```python
from build123d import *

# Parameters (mm, degrees)
SKETCH1_R           = 0.9
SKETCH1_R_2         = 0.65
BOSS_EXTRUDE1_DEPTH = 220
SKETCH2_R           = 0.9
SKETCH2_R_2         = 0.65
CUT_EXTRUDE1_DEPTH  = 6
SKETCH1_3_R         = 0.65
BOSS_EXTRUDE2_DEPTH = 5
FILLET1_R           = 3
FILLET2_R           = 1


with BuildPart() as part:
    # Sketch1 → Boss-Extrude1 (new body)
    # profile 1 of 7: a face of its own
    with BuildSketch(Plane(origin=(-29.212578399, 0, 0), x_dir=(0, 0, -1), z_dir=(1, 0, 0))):
        with BuildLine():
            ThreePointArc((7.945170891, 34.240487163), (7.203959388, 34.412879785), (6.445170891, 34.470791156))
            Line((6.445170891, 34.470791156), (4.445170891, 34.470791156))
            Line((4.445170891, 34.470791156), (4.445170891, 27.470791156))
            Line((4.445170891, 27.470791156), (11.445170891, 27.470791156))
            Line((11.445170891, 27.470791156), (11.445170891, 29.470791156))
            ThreePointArc((11.445170891, 29.470791156), (11.38725952, 30.229579652), (11.214866898, 30.970791156))
            Line((11.214866898, 30.970791156), (7.945170891, 30.970791156))
            Line((7.945170891, 30.970791156), (7.945170891, 34.240487163))
        make_face()
        with Locations((9.695170891, 29.220791156)):
            Circle(SKETCH1_R, mode=Mode.SUBTRACT)
        with Locations((6.195170891, 32.720791156)):
            Circle(SKETCH1_R, mode=Mode.SUBTRACT)
    # profile 2 of 7: a face of its own
    with BuildSketch(Plane(origin=(-29.212578399, 0, 0), x_dir=(0, 0, -1), z_dir=(1, 0, 0))):
        with BuildLine():
            Line((11.445170891, 29.470791156), (11.445170891, 30.970791156))
            Line((11.445170891, 30.970791156), (11.214866898, 30.970791156))
            ThreePointArc((11.214866898, 30.970791156), (11.38725952, 30.229579652), (11.445170891, 29.470791156))
        make_face()
    # profile 3 of 7: a face of its own
    with BuildSketch(Plane(origin=(-29.212578399, 0, 0), x_dir=(0, 0, -1), z_dir=(1, 0, 0))):
        with BuildLine():
            Line((7.945170891, 34.240487163), (7.945170891, 34.470791156))
            Line((7.945170891, 34.470791156), (6.445170891, 34.470791156))
            ThreePointArc((6.445170891, 34.470791156), (7.203959388, 34.412879785), (7.945170891, 34.240487163))
        make_face()
    # profile 4 of 7: a face of its own
    with BuildSketch(Plane(origin=(-29.212578399, 0, 0), x_dir=(0, 0, -1), z_dir=(1, 0, 0))):
        with Locations((6.195170891, 32.720791156)):
            Circle(SKETCH1_R)
        with Locations((6.195170891, 32.720791156)):
            Circle(SKETCH1_R_2, mode=Mode.SUBTRACT)
    # profile 5 of 7: a face of its own
    with BuildSketch(Plane(origin=(-29.212578399, 0, 0), x_dir=(0, 0, -1), z_dir=(1, 0, 0))):
        with Locations((6.195170891, 32.720791156)):
            Circle(SKETCH1_R_2)
    # profile 6 of 7: a face of its own
    with BuildSketch(Plane(origin=(-29.212578399, 0, 0), x_dir=(0, 0, -1), z_dir=(1, 0, 0))):
        with Locations((9.695170891, 29.220791156)):
            Circle(SKETCH1_R)
        with Locations((9.695170891, 29.220791156)):
            Circle(SKETCH1_R_2, mode=Mode.SUBTRACT)
    # profile 7 of 7: a face of its own
    with BuildSketch(Plane(origin=(-29.212578399, 0, 0), x_dir=(0, 0, -1), z_dir=(1, 0, 0))):
        with Locations((9.695170891, 29.220791156)):
            Circle(SKETCH1_R_2)
    extrude(amount=BOSS_EXTRUDE1_DEPTH)

    # Sketch2 → Cut-Extrude1 (cut)
    # profile 1 of 4: a face of its own
    with BuildSketch(Plane(origin=(190.787421601, 0, 0), x_dir=(0, 0, -1), z_dir=(1, 0, 0))):
        with Locations((6.195170891, 32.720791156)):
            Circle(SKETCH2_R)
        with Locations((6.195170891, 32.720791156)):
            Circle(SKETCH2_R_2, mode=Mode.SUBTRACT)
    # profile 2 of 4: a face of its own
    with BuildSketch(Plane(origin=(190.787421601, 0, 0), x_dir=(0, 0, -1), z_dir=(1, 0, 0))):
        with Locations((6.195170891, 32.720791156)):
            Circle(SKETCH2_R_2)
    # profile 3 of 4: a face of its own
    with BuildSketch(Plane(origin=(190.787421601, 0, 0), x_dir=(0, 0, -1), z_dir=(1, 0, 0))):
        with Locations((9.695170891, 29.220791156)):
            Circle(SKETCH2_R)
        with Locations((9.695170891, 29.220791156)):
            Circle(SKETCH2_R_2, mode=Mode.SUBTRACT)
    # profile 4 of 4: a face of its own
    with BuildSketch(Plane(origin=(190.787421601, 0, 0), x_dir=(0, 0, -1), z_dir=(1, 0, 0))):
        with Locations((9.695170891, 29.220791156)):
            Circle(SKETCH2_R_2)
    extrude(amount=-CUT_EXTRUDE1_DEPTH, mode=Mode.SUBTRACT)

    # Sketch1_3 → Boss-Extrude2 (add)
    with BuildSketch(Plane(origin=(-29.212578399, 0, 0), x_dir=(0, 0, -1), z_dir=(1, 0, 0))):
        with Locations((6.195170891, 32.720791156)):
            Circle(SKETCH1_3_R)
        with Locations((9.695170891, 29.220791156)):
            Circle(SKETCH1_3_R)
    extrude(amount=-BOSS_EXTRUDE2_DEPTH)

    # Fillet1
    fillet1_edges = [part.edges().sort_by_distance(p)[0] for p in [
        (80.787421601, 27.470791156, -4.445170891),
    ]]
    fillet(fillet1_edges, radius=FILLET1_R)

    # Fillet2
    fillet2_edges = [part.edges().sort_by_distance(p)[0] for p in [
        (80.787421601, 30.970791156, -11.445170891),
        (80.787421601, 34.470791156, -7.945170891),
    ]]
    fillet(fillet2_edges, radius=FILLET2_R)


solid = part.part
```
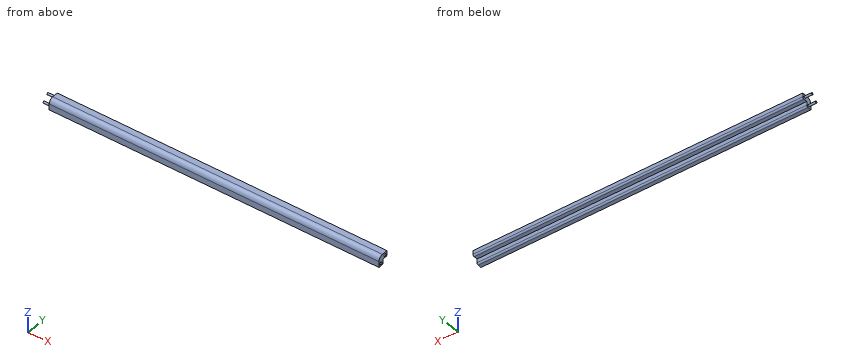
Could you check a few things on this model? Use its own coordinates, in mm. Round coordinates to 2 decimals unless told otherwise and drop trailing zeros. Loops run counter-clockwise (first coordinate to the right, second up) from the corner with the lowest first, then second, coordinate; pieces in that order, holes last. Notation, with made-up numbers: (-39, 24.25) - (2, 24.25) arc R14 cw to (2, 51.25) - close; hole circle Ø2 at (47, -18). An arc over 180 degrees is marked (long way). Answer in a Markdown table with one row per item. Add a question column.
(1) I need wall thicknesses on line 1 along Z through (x, y) = (144, 33); line 2 along X through (y, z) = (29.5, -9.25); line 3 along Y through (x, z) = (57, -10.25). Which ranges of each line are inside material? Lowest first, please.
(2) If we section it at A-A (x = 1.5): Please give me the cut outline in (y, z).
(3) I'm going to push flat-ended pins straight in: pin 1 (2 mm diameter, centred on y = 32.72, z = -6.2, fed in from +X); pin 2 (2.5 mm diameter, centred on x = 64, y = 32.5, fed in from -Z); pin 3 (2 mm diameter, centred on x = 63.5, z = -8.5, fed in from +Y); pin 4 (0.9 mm diameter, centred on y = 29.5, z = -10, fed in from +X). Where does each tip first touch, or does it pass through?
Model answer:
| question | item | result |
|---|---|---|
| 1 | line 1 | z = -7.95 to -4.45 |
| 1 | line 2 | x = -34.21 to 184.79 |
| 1 | line 3 | y = 27.47 to 30.97 |
| 2 | outline | (27.47, -11.45) - (29.97, -11.45) arc R1 ccw to (30.97, -10.45) - (30.97, -7.95) - (33.47, -7.95) arc R1 ccw to (34.47, -6.95) - (34.47, -4.45) - (30.47, -4.45) arc R3 ccw to (27.47, -7.45) - close |
| 3 | pin 1 | stops at x = 190.79 |
| 3 | pin 2 | stops at z = -7.95 |
| 3 | pin 3 | stops at y = 34.3 |
| 3 | pin 4 | stops at x = 184.79 |
